Could you check a few things on this model? Use its own coordinates, in mm. A direction names the side the tool comes from. Coordinates: 2 decimals unless noted, no trailing zeros. Order: outer loops, then holes, each group sorted by start corner. A loop starts at its lowest first (then second) coordinate and runs counter-clockwise, first axis right, second up.
```python
from build123d import *

# Parameters (mm, degrees)
SKETCH1_W                      = 113.7412
SKETCH1_H                      = 72.517
BOSS_EXTRUDE1_DEPTH            = 9.525
BOSS_EXTRUDE5_START            = -38.1
BOSS_EXTRUDE5_DEPTH            = 76.2
CUT_EXTRUDE3_REACH             = 88.637
SKETCH1_6_R                    = 3.37
CUT_EXTRUDE3_DIRECTION_2_DEPTH = 87.637123003
BOSS_EXTRUDE6_DEPTH            = 22.225
SKETCH7_R                      = 2.4892
CUT_EXTRUDE4_DEPTH             = 92.543856508
SKETCH8_R                      = 3.429
CUT_EXTRUDE5_DEPTH             = 5.08
CUT_EXTRUDE7_DEPTH             = 6.35
FILLET2_R                      = 0.79375


# Read off the part's stored shape, not the designer's step: Boss-Extrude5
with BuildPart() as part:
    # Sketch1 → Boss-Extrude1 (new, symmetric)
    with BuildSketch(Plane.XY):
        Rectangle(SKETCH1_W, SKETCH1_H)
    extrude(amount=BOSS_EXTRUDE1_DEPTH, both=True)

    # Boss-Extrude5 outline → Boss-Extrude5 (add)
    with BuildSketch(Plane(origin=(0, 0, 0), x_dir=(0, 0, -1), z_dir=(1, 0, 0)).offset(BOSS_EXTRUDE5_START)):
        Polygon((54.378737717, -12.40934461), (48.41644887, -1.195910181), (9.525, -21.874860356), (9.525, -36.2585), align=None)
    extrude(amount=BOSS_EXTRUDE5_DEPTH)

    # Sketch1<6> → Cut-Extrude3 (cut, up to next)
    with BuildSketch(Plane.XY, mode=Mode.PRIVATE) as cut_extrude3_sk1:
        with Locations(Location((-28.8925, 0, 0), (0, 0, 180))):
            Circle(SKETCH1_6_R)
    cut_extrude3_tool1 = extrude(cut_extrude3_sk1.sketch, amount=-CUT_EXTRUDE3_REACH, mode=Mode.PRIVATE) & part.part
    # Sketch1<6> → Cut-Extrude3 (cut, up to next)
    with BuildSketch(Plane.XY, mode=Mode.PRIVATE) as cut_extrude3_sk2:
        with Locations(Location((28.8925, 0, 0), (0, 0, 180))):
            Circle(SKETCH1_6_R)
    cut_extrude3_tool2 = extrude(cut_extrude3_sk2.sketch, amount=-CUT_EXTRUDE3_REACH, mode=Mode.PRIVATE) & part.part
    add(cut_extrude3_tool1.solids().sort_by_distance((-28.8925, 0, 0))[0], mode=Mode.SUBTRACT)
    add(cut_extrude3_tool2.solids().sort_by_distance((28.8925, 0, 0))[0], mode=Mode.SUBTRACT)

    # Sketch1<6> → Cut-Extrude3 direction 2 (cut)
    with BuildSketch(Plane.XY):
        with Locations(Location((-28.8925, 0, 0), (0, 0, 180))):
            Circle(SKETCH1_6_R)
        with Locations(Location((28.8925, 0, 0), (0, 0, 180))):
            Circle(SKETCH1_6_R)
    extrude(amount=CUT_EXTRUDE3_DIRECTION_2_DEPTH, mode=Mode.SUBTRACT)

    # Sketch6 → Boss-Extrude6 (add, symmetric)
    with BuildSketch(Plane(origin=(0, 0, 0), x_dir=(0, 0, -1), z_dir=(1, 0, 0))):
        Polygon((9.525, 36.2585), (9.525, -21.874860356), (48.41644887, -1.195910181), align=None)
    extrude(amount=BOSS_EXTRUDE6_DEPTH, both=True)

    # Sketch7 → Cut-Extrude4 (cut, through all)
    with BuildSketch(Plane(origin=(0, -21.001854955, -11.166884362), x_dir=(1, 0, 0), z_dir=(0, 0.882947592858928, 0.46947156278588875))):
        with Locations(Location((31.75, 35.837741163, 0), (0, 0, 270))):
            Circle(SKETCH7_R)
        with Locations(Location((31.75, 16.787741163, 0), (0, 0, 270))):
            Circle(SKETCH7_R)
        with Locations(Location((-31.75, 35.837741163, 0), (0, 0, 270))):
            Circle(SKETCH7_R)
        with Locations(Location((-31.75, 16.787741163, 0), (0, 0, 270))):
            Circle(SKETCH7_R)
    extrude(amount=-CUT_EXTRUDE4_DEPTH, mode=Mode.SUBTRACT)

    # Sketch8 → Cut-Extrude5 (cut)
    with BuildSketch(Plane.XY.offset(9.525)):
        with Locations((-14, 14)):
            Circle(SKETCH8_R)
        with Locations((14, 14)):
            Circle(SKETCH8_R)
        with Locations((-14, -14)):
            Circle(SKETCH8_R)
        with Locations((14, -14)):
            Circle(SKETCH8_R)
    extrude(amount=-CUT_EXTRUDE5_DEPTH, mode=Mode.SUBTRACT)

    # Sketch11 → Cut-Extrude7 (cut)
    with BuildSketch(Plane(origin=(22.225, 0, 0), x_dir=(0, 0, -1), z_dir=(1, 0, 0))):
        Polygon((9.525, 3.37), (9.525, -3.37), (9.525, -8.1325), (15.875, -8.1325), (15.875, 8.1325), (9.525, 8.1325), align=None)
    cut_extrude7 = extrude(amount=-CUT_EXTRUDE7_DEPTH, mode=Mode.SUBTRACT)

    # Mirror1: Cut-Extrude7 across plane
    add(cut_extrude7.mirror(Plane(origin=(0, 0, 0), x_dir=(0, 0, 1), z_dir=(1, 0, 0))), mode=Mode.SUBTRACT)

    # Fillet2
    fillet2_edges = [part.edges().sort_by_distance(p)[0] for p in [
        (19.05, 8.1325, -15.875),
        (19.05, -8.1325, -15.875),
        (-19.05, -8.1325, -15.875),
        (-19.05, 8.1325, -15.875),
    ]]
    fillet(fillet2_edges, radius=FILLET2_R)


solid = part.part
```
Item 1: Suppose I cut it at C-C (y = 5). List the corners of the cut face in (x, z) for me (3 decimals), and give its area (3 significant figures).
Item 2: Thinking about a two-plate mould opening in Z: for faces 5 (the face through (14, 14, 4.445)), 6 (the face through (-56.871, -1, 0)), 7 (the face through (-19, -8.132, -12)), 8 (the face through (-15.875, 0, -13)), which applies, +Z half, -Z half, draft (parallel to the pull), parting line (faces both ways), or undercut?
Item 3: I need wall thicknesses on line 1 (Y direction, x = -14, z = 5.8); line 2 (X direction, y = 12.5, z = -14.5) (3 decimals); line 3 (Z direction, x = 23.5, y = 9) (3 decimals). Which ranges of each line are inside material? Lowest first, please.
Item 4: For pin 1 Ø3 at (x, y) = (44, -23.5) entering from -Z (3 decimals); pin 2 Ø4 at (x, y) = (14, 14) entering from +Z (3 decimals); pin 3 Ø11.5 at (y, z) = (-6.5, -35.5) entering from +X, each with a flat end and sliding along its axis, tell me the tip position at first contact or that it passes through.
Item 5: Suppose I cut it at D-D (x = -14). List the corners of the cut face in (y, z) for me (1 decimal), and give its area (3 significant figures).
Item 6: Suppose I cut it at B-B (z = -38). List the corners of the cut face in (x, y) for me (3 decimals).
Item 7: Which directions (+Z, -Z, +X, -X, +Y, -Y) give clear straight access to the entire face, cutting with the end or side of a thin tool? Please do faces 1 (the face through (-22.225, 8, -24)), 2 (the face through (-17.426, -13.849, 7.021)), 3 (the face through (-19, 0, -15.875)), 4 (the face through (22.225, 8, -24)).
Item 8: Suppose I cut it at A-A (x = 24). List the corners of the cut face in (y, z) for me (1 decimal), and give its area (3 significant figures).
Geometry results:
1. outline: (-56.871, -9.525) - (-15.875, -9.525) - (-15.875, -15.875) - (-22.225, -15.875) - (-22.225, -41.983) - (22.225, -41.983) - (22.225, -15.875) - (15.875, -15.875) - (15.875, -9.525) - (56.871, -9.525) - (56.871, 9.525) - (-56.871, 9.525) - close
1. area: 3,530 mm2
2. face 5: +Z half
2. face 6: draft
2. face 7: undercut
2. face 8: undercut
3. line 1: y = -36.26 to -17.43, -10.57 to 10.57, 17.43 to 36.26
3. line 2: x = -22.225 to 22.225
3. line 3: z = -9.525 to 9.525
4. pin 1: stops at z = -9.525
4. pin 2: stops at z = 4.445
4. pin 3: stops at x = 38.1
5. outline: (-36.3, -9.5) - (-12.4, -54.4) - (-1.2, -48.4) - (36.3, -9.5) - (36.3, 9.5) - (17.4, 9.5) - (17.4, 4.4) - (10.6, 4.4) - (10.6, 9.5) - (-10.6, 9.5) - (-10.6, 4.4) - (-17.4, 4.4) - (-17.4, 9.5) - (-36.3, 9.5) - close
5. area: 3,040 mm2
6. outline: (-38.1, -21.118) - (38.1, -21.118) - (38.1, -6.734) - (22.225, -6.734) - (22.225, 8.836) - (-22.225, 8.836) - (-22.225, -6.734) - (-38.1, -6.734) - close
7. face 1: -X, +Y
7. face 2: +Z
7. face 3: -X
7. face 4: +X, +Y
8. outline: (-36.3, -9.5) - (-12.4, -54.4) - (-1.2, -48.4) - (-21.9, -9.5) - (36.3, -9.5) - (36.3, 9.5) - (-36.3, 9.5) - close
8. area: 1,980 mm2
